Could you check a few things on this model? Use its own coordinates, in mm. Face numbers are marked on the shaded views. A direction names the side the tool comes from. Coordinates: 2 decimals unless noted, no trailing zeros. Order: outer loops, then holes, each group sorted by start corner. A loop starts at its lowest first (then second) coordinate and runs counter-clockwise, first axis right, second up. Notation, with made-up numbers: (63.25, 43) -> (68.25, 43) arc R18 ccw to (68.25, 61) -> close; hole circle Ø10 at (79.5, -15.5). An arc over 180 degrees is marked (long way). Return JSON: item names as keys, results as strings. Group by question number.
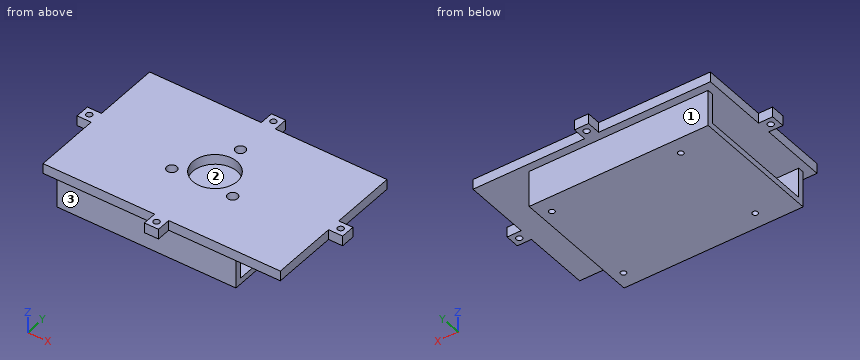
from build123d import *

# Parameters (mm, degrees)
CROQUIS1_R                  = 1.5
SALIENTE_EXTRUIR1_DEPTH     = 5
CROQUIS3_R                  = 11
CROQUIS3_R_2                = 2.5
CORTAR_EXTRUIR1_DEPTH       = 10
CROQUIS4_W                  = 89
CROQUIS4_H                  = 65
CROQUIS4_W_2                = 83
CROQUIS4_H_2                = 59
SALIENTE_EXTRUIR3_DEPTH     = 18
CROQUIS5_W                  = 83
CROQUIS5_H                  = 59
CROQUIS5_R                  = 1.375
SALIENTE_EXTRUIR4_DEPTH     = 3
SALIENTE_EXTRUIR5_START     = -89
SALIENTE_EXTRUIR5_OUTLINE_W = 15
SALIENTE_EXTRUIR5_OUTLINE_H = 59
SALIENTE_EXTRUIR5_DEPTH     = 89


# Read off the part's stored shape, not the designer's step: Saliente-Extruir5
with BuildPart() as part:
    # Croquis1 → Saliente-Extruir1 (new body)
    with BuildSketch(Plane.XY):
        Polygon((-40.689655172, 34.755747126), (14.810344828, 34.755747126), (14.810344828, 41.755747126), (21.810344828, 41.755747126), (21.810344828, 34.755747126), (77.310344828, 34.755747126), (77.310344828, 1.755747126), (84.310344828, 1.755747126), (84.310344828, -5.244252874), (77.310344828, -5.244252874), (77.310344828, -38.244252874), (21.810344828, -38.244252874), (21.810344828, -45.244252874), (14.810344828, -45.244252874), (14.810344828, -38.244252874), (-40.689655172, -38.244252874), (-40.689655172, -5.244252874), (-47.689655172, -5.244252874), (-47.689655172, 1.755747126), (-40.689655172, 1.755747126), align=None)
        with Locations((18.310344828, 38.255747126)):
            Circle(CROQUIS1_R, mode=Mode.SUBTRACT)
        with Locations((-44.189655172, -1.744252874)):
            Circle(CROQUIS1_R, mode=Mode.SUBTRACT)
        with Locations((80.810344828, -1.744252874)):
            Circle(CROQUIS1_R, mode=Mode.SUBTRACT)
        with Locations((18.310344828, -41.744252874)):
            Circle(CROQUIS1_R, mode=Mode.SUBTRACT)
    extrude(amount=-SALIENTE_EXTRUIR1_DEPTH)

    # Croquis3 → Cortar-Extruir1 (cut)
    with BuildSketch(Plane(origin=(0, 0, -5), x_dir=(-1, 0, 0), z_dir=(0, 0, -1))):
        with Locations((-18.310344828, -1.744252874)):
            Circle(CROQUIS3_R)
        with Locations((-18.310344828, 15.700747126)):
            Circle(CROQUIS3_R_2)
        with Locations((-3.198201532, -10.469252874)):
            Circle(CROQUIS3_R_2)
        with Locations((-33.422488124, -10.469252874)):
            Circle(CROQUIS3_R_2)
    extrude(amount=-CORTAR_EXTRUIR1_DEPTH, mode=Mode.SUBTRACT)

    # Croquis4 → Saliente-Extruir3 (add)
    with BuildSketch(Plane(origin=(0, 0, -5), x_dir=(-1, 0, 0), z_dir=(0, 0, -1))):
        with Locations((-7.810344828, -1.744252874)):
            Rectangle(CROQUIS4_W, CROQUIS4_H)
        with Locations((-7.810344828, -1.744252874)):
            Rectangle(CROQUIS4_W_2, CROQUIS4_H_2, mode=Mode.SUBTRACT)
    extrude(amount=SALIENTE_EXTRUIR3_DEPTH)

    # Croquis5 → Saliente-Extruir4 (add)
    with BuildSketch(Plane(origin=(0, 0, -23), x_dir=(-1, 0, 0), z_dir=(0, 0, -1))):
        with Locations((-7.810344828, -1.744252874)):
            Rectangle(CROQUIS5_W, CROQUIS5_H)
        with Locations((-46.810344828, 22.755747126)):
            Circle(CROQUIS5_R, mode=Mode.SUBTRACT)
        with Locations((-46.810344828, -26.244252874)):
            Circle(CROQUIS5_R, mode=Mode.SUBTRACT)
        with Locations((17.312228898, 22.755747126)):
            Circle(CROQUIS5_R, mode=Mode.SUBTRACT)
        with Locations((18.687228898, -26.244252874)):
            Circle(CROQUIS5_R, mode=Mode.SUBTRACT)
    extrude(amount=-SALIENTE_EXTRUIR4_DEPTH)

    # Saliente-Extruir5 outline → Saliente-Extruir5 (cut)
    with BuildSketch(Plane(origin=(52.310344828, 0, 0), x_dir=(0, 0, -1), z_dir=(1, 0, 0)).offset(SALIENTE_EXTRUIR5_START)):
        with Locations((12.5, -1.744252874)):
            Rectangle(SALIENTE_EXTRUIR5_OUTLINE_W, SALIENTE_EXTRUIR5_OUTLINE_H)
    extrude(amount=SALIENTE_EXTRUIR5_DEPTH, mode=Mode.SUBTRACT)


solid = part.part
Q1. I want a section at A-A on x = -8. Please give me the cut outline in (y, z).
Q2. I need wall thicknesses on line 1 along Z through (x, y) = (37, 3); line 2 along Y through (x, z) = (38, -8.5); line 3 along Z through (x, y) = (57, 5). Which ranges of each line are inside material? Lowest first, please. Write a range as from..to.
Q3. On a 3-axis mill with a long thin cutter (end or side, diameter ignored), from which of +Z, -Z, +X, -X, +Y, -Y can I reach the whole of each face in a straight line? I mean the marked faces 1, 2 and 3. Say none if no direction works.
Q4. I want a section at C-C on z = -9. Please give me the cut outline in (x, y).
Q5. I want a section at D-D on y = 6.5. Please give me the cut outline in (x, z), and give its area (3 significant figures).
Q6. I'm going to push flat-ended pins straight in: pin 1 Ø1.5 at (y, z) = (-21.5, -3.5) entering from -X; pin 2 Ø2 at (x, z) = (-13, -6.5) entering from -Y; pin 3 Ø6 at (x, z) = (34.5, -14.5) entering from +Y; pin 4 Ø12 at (x, y) = (35.5, -23.5) entering from +Z. Where does each tip first touch, or does it pass through?
Q7. I want a section at B-B on y = -17.5. Please give me the cut outline in (x, z), and give its area (3 significant figures).
Response values:
{
 "1": {"outline": "(-38.24, -5) -> (-34.24, -5) -> (-34.24, -23) -> (30.76, -23) -> (30.76, -5) -> (34.76, -5) -> (34.76, 0) -> (-38.24, 0) -> close; hole (-31.24, -20) -> (27.76, -20) -> (27.76, -5) -> (-31.24, -5) -> close"},
 "2": {"line 1": "z = -23..-20, -5..0", "line 2": "y = -34.24..-31.24, 27.76..30.76", "line 3": "z = -5..0"},
 "3": {"face 1": "-Z, +X, -X, +Y", "face 2": "+X, -X", "face 3": "-Z, +X, -X, -Y"},
 "4": {"outline": "(-36.69, -34.24) -> (52.31, -34.24) -> (52.31, -31.24) -> (-36.69, -31.24) -> close; (-36.69, 27.76) -> (52.31, 27.76) -> (52.31, 30.76) -> (-36.69, 30.76) -> close"},
 "5": {"outline": "(-40.69, -5) -> (11.03, -5) -> (11.03, 0) -> (-40.69, 0) -> close; (-36.69, -23) -> (52.31, -23) -> (52.31, -20) -> (-36.69, -20) -> close; (25.59, -5) -> (77.31, -5) -> (77.31, 0) -> (25.59, 0) -> close", "area": "784 mm²"},
 "6": {"pin 1": "stops at x = -40.69", "pin 2": "stops at y = -34.24", "pin 3": "stops at y = 30.76", "pin 4": "stops at z = 0"},
 "7": {"outline": "(-40.69, -5) -> (77.31, -5) -> (77.31, 0) -> (-40.69, 0) -> close; (-36.69, -23) -> (52.31, -23) -> (52.31, -20) -> (-36.69, -20) -> close", "area": "857 mm²"}
}
